Autodesk Fusion 360 part; units mm, degrees
sketch "Sketch1" plane through (0, 0, 0) normal (1, 0, 0) x (0, 1, 0)
  line L0 (0, -5.7569) -> (0, 10)
  line L1 (0, 10) -> (14.2431, 10)
  line L2 (14.2431, 10) -> (14.2431, 50)
  line L3 (14.2431, 50) -> (30, 50)
  line L4 (30, 30) -> (50, 30)
  line L5 (50, 30) -> (50, 50)
  line L6 (50, 50) -> (65.7569, 50)
  line L7 (25, -25) -> (23.7742, -25.0601)
  line L8 (65.7569, 50) -> (65.7569, 10)
  line L9 (65.7569, 10) -> (80, 10)
  line L10 (80, 10) -> (80, 0)
  line L11 (0, -5.7569) -> (0, 0)
  line L12 (30, 50) -> (30, 30)
  line L13 (30, 20) -> (50, 20)
  line L14 (50, 20) -> (50, 0)
  line L15 (30, 20) -> (30, 0)
  line L16 (80, 0) -> (50, 0)
  line L17 (30, 0) -> (0, 0)
  dimension "d1" = 10
  dimension "d2" = 80
  dimension "d3" = 20
  dimension "d4" = 15.7569
  dimension "d5" = 50
  dimension "d6" = 10
  dimension "d7" = 30
extrude "Extrude1" add sketch "Sketch1" along normal blind 10
Input: part model. Units: mm. Frame: model coordinates. A direction names the side the tool comes from. Coordinates: 2 decimals unless noted, no trailing zeros. Loops run counter-clockwise (first coordinate to the right, second up) from the corner with the lowest first, then second, coordinate; pieces in that order, holes last. Notation, with made-up numbers: M -27.75,49.25 L -3.75,49.25 A20 cw -3.75,80.25 Z; hole C 48,-37.5 d6. An arc over 180 degrees is marked long. One line per item, written item: value.
(1) Section B-B (x = 2). Output: boundary loops of the cut face in (y, z), and give its area (3 significant figures).
Filled in:
outline: M 0,0 L 30,0 L 30,20 L 50,20 L 50,0 L 80,0 L 80,10 L 65.76,10 L 65.76,50 L 50,50 L 50,30 L 30,30 L 30,50 L 14.24,50 L 14.24,10 L 0,10 Z
area: 2,060 mm^2
(2) Line query: line 1 along Y through (x, z) = (2, 5); line 2 along Y through (x, z) = (1.5, 11); line 3 along Z through (x, y) = (1, 7.5). Output: solid intervals per line, ascending. Write a range as from..to.
Filled in:
line 1: 0..30, 50..80
line 2: 14.24..30, 50..65.76
line 3: 0..10
(3) Pin query (flat end, axial travel): pin 1 (5 mm diameter, centred on x = 5, z = 27, fed in from +Y); pin 2 (6 mm diameter, centred on y = 71, z = 11.5, fed in from -X); pin 3 (3 mm diameter, centred on x = 3, z = 43, fed in from -Y); pin 4 (3 mm diameter, centred on x = 5, y = 43, fed in from +Z). Return the tip coordinate at first contact, or that it passes through.
Filled in:
pin 1: y = 65.76
pin 2: x = 0
pin 3: y = 14.24
pin 4: z = 30
(4) Reachability of faces 4 (the flat face through (5, 7, 10)), 5 (the flat face through (5, 50, 10)), 6 (the flat face through (5, 50, 40)), 7 (the flat face through (5, 73, 10)) from +Z, -Z, +X, -X, +Y, -Y: full face, straight path, thin tool, end or side. Return the list, or none.
Filled in:
face 4: +Z, +X, -X, -Y
face 5: -Z, +X, -X
face 6: +Z, +X, -X
face 7: +Z, +X, -X, +Y
(5) Section C-C (z = 6). Output: boundary loops of the cut face in (x, y).
Filled in:
outline: M 0,0 L 10,0 L 10,30 L 0,30 Z; M 0,50 L 10,50 L 10,80 L 0,80 Z
(6) Section A-A (z = 15.5). Output: boundary loops of the cut face in (x, y).
Filled in:
outline: M 0,14.24 L 10,14.24 L 10,30 L 0,30 Z; M 0,50 L 10,50 L 10,65.76 L 0,65.76 Z
(7) Pull-direction query (Y, two-part tool) for faces 1 (the flat face through (5, 40, 20)), 2 (the flat face through (5, 14.243, 30)), 3 (the flat face through (0, 40, 21)); classes: +Y half, -Y half, draft (parallel to the pull), parting line (faces both ways), or undercut.
Filled in:
face 1: undercut
face 2: -Y half
face 3: draft
(8) Section D-D (y = 42). Output: boundary loops of the cut face in (x, z), and give its area (3 significant figures).
Filled in:
outline: M 0,20 L 10,20 L 10,30 L 0,30 Z
area: 100 mm^2
